Model file for the job. Use its own axes, mm. A direction names the side the tool comes from. Coordinates: 2 decimals unless noted, no trailing zeros. Order: outer loops, then holes, each group sorted by start corner. A loop starts at its lowest first (then second) coordinate and runs counter-clockwise, first axis right, second up.
from build123d import *

# Parameters (mm, degrees)
SKETCH_1_R      = 1.1
EXTRUDE_1_DEPTH = 3
EXTRUDE_2_DEPTH = 2


with BuildPart() as part:
    # 草图1 → 凸台-拉伸1 (new body)
    with BuildSketch(Plane.XY):
        with BuildLine():
            Line((-5, 5.5), (5, 5.5))
            ThreePointArc((5, 5.5), (10.5, 0), (5, -5.5))
            Line((5, -5.5), (-5, -5.5))
            ThreePointArc((-5, -5.5), (-10.5, 0), (-5, 5.5))
        make_face()
        Circle(SKETCH_1_R, mode=Mode.SUBTRACT)
    extrude(amount=EXTRUDE_1_DEPTH)

    # 草图3 → 凸台-拉伸2 (add)
    with BuildSketch(Plane(origin=(0, 0, 0), x_dir=(-1, 0, 0), z_dir=(0, 0, -1))):
        with BuildLine():
            Line((-1.802775638, 3), (-6.873863542, 3))
            ThreePointArc((-6.873863542, 3), (-7.154882442, 2.248923573), (-7.354101966, 1.472135955))
            Line((-7.354101966, 1.472135955), (-7.354101966, 1))
            Line((-7.354101966, 1), (-3.354101966, 1))
            ThreePointArc((-3.354101966, 1), (-2.765564437, 2.145146462), (-1.802775638, 3))
        make_face()
        with BuildLine():
            Line((-7.354101966, -1.472135955), (-7.354101966, -1))
            Line((-7.354101966, -1), (-3.354101966, -1))
            ThreePointArc((-3.354101966, -1), (-2.765564437, -2.145146462), (-1.802775638, -3))
            Line((-1.802775638, -3), (-6.873863542, -3))
            ThreePointArc((-6.873863542, -3), (-7.154882442, -2.248923573), (-7.354101966, -1.472135955))
        make_face()
        with BuildLine():
            Line((1.802775638, -3), (6.873863542, -3))
            ThreePointArc((6.873863542, -3), (7.154882442, -2.248923573), (7.354101966, -1.472135955))
            Line((7.354101966, -1.472135955), (7.354101966, -1))
            Line((7.354101966, -1), (3.354101966, -1))
            ThreePointArc((3.354101966, -1), (2.765564437, -2.145146462), (1.802775638, -3))
        make_face()
        with BuildLine():
            Line((7.354101966, 1.472135955), (7.354101966, 1))
            Line((7.354101966, 1), (3.354101966, 1))
            ThreePointArc((3.354101966, 1), (2.765564437, 2.145146462), (1.802775638, 3))
            Line((1.802775638, 3), (6.873863542, 3))
            ThreePointArc((6.873863542, 3), (7.154882442, 2.248923573), (7.354101966, 1.472135955))
        make_face()
    extrude(amount=EXTRUDE_2_DEPTH)


solid = part.part
Q1. Mould opens along X. For faces 1 (the face through (1.05, 0.33, 1.48)), 2 (the face through (2.8, 2.1, -1)), 3 (the face through (-10.5, -0.1, 1.5)), 4 (the face through (-5, -2, -2)) say: pulls with the +X half, pulls with the -X half, needs draft (parallel to the pull), parting line crosses it, or undercut.
Established:
face 1: undercut
face 2: undercut
face 3: pulls with the -X half
face 4: needs draft
Q2. Probe line 1 (Y direction, x = 4.75, z = -0.9); line 2 (Y direction, x = 0, z = 2.1); line 3 (Z direction, x = 1, y = 1.75). List the from-to ranges inside material, lowest first.
Established:
line 1: y = -3 to -1, 1 to 3
line 2: y = -5.5 to -1.1, 1.1 to 5.5
line 3: z = 0 to 3
Q3. Cut at D-D, the plane z = -0.55. List the corners of the cut face in (x, y).
Established:
outline: (-7.35, -1.47) arc R7.5 ccw to (-6.87, -3) - (-1.8, -3) arc R3.5 cw to (-3.35, -1) - (-7.35, -1) - close; (-7.35, 1) - (-3.35, 1) arc R3.5 cw to (-1.8, 3) - (-6.87, 3) arc R7.5 ccw to (-7.35, 1.47) - close; (1.8, -3) - (6.87, -3) arc R7.5 ccw to (7.35, -1.47) - (7.35, -1) - (3.35, -1) arc R3.5 cw to start; (1.8, 3) arc R3.5 cw to (3.35, 1) - (7.35, 1) - (7.35, 1.47) arc R7.5 ccw to (6.87, 3) - close
Q4. Cut at B-B, the plane x = 4.5. List the corners of the cut face in (y, z).
Established:
outline: (-5.5, 0) - (-3, 0) - (-3, -2) - (-1, -2) - (-1, 0) - (1, 0) - (1, -2) - (3, -2) - (3, 0) - (5.5, 0) - (5.5, 3) - (-5.5, 3) - close
Q5. Cut at C-C, the plane y = 0. List the corners of the cut face in (x, z), plus the area to 3 significant figures.
Established:
outline: (-10.5, 0) - (-1.1, 0) - (-1.1, 3) - (-10.5, 3) - close; (1.1, 0) - (10.5, 0) - (10.5, 3) - (1.1, 3) - close
area: 56.4 mm2
Q6. Which spindle directions (+Z, -Z, +X, -X, +Y, -Y) get a long thin tool onto all of the face, cutting with end or side? Do faces 5 (the face through (4, -3, -1)), 6 (the face through (-2.8, -2.1, -1)), 7 (the face through (7.15, -2.26, -0.99)), 8 (the face through (4, 3, -1)), 9 (the face through (-5, -1, -1)). Say none if no direction does.
Established:
face 5: -Z, +X, -X, -Y
face 6: -Z
face 7: -Z, +X, -Y
face 8: -Z, +X, -X, +Y
face 9: -Z, +X, -X
Q7. Drop flat-ended pins along their axis: P1, Ø1.6, axis at x = -5.5, z = -1, coming from the -Y side; P2, Ø0.6, axis at x = 5, z = -1.5, coming from the +Y side. Give the stop position or say it passes through.
Established:
P1: stops at y = -3
P2: stops at y = 3
Q8. Cut at A-A, the plane z = 1.45. List the corners of the cut face in (x, y), plus the area to 3 significant figures.
Established:
outline: (-5, -5.5) - (5, -5.5) arc R5.5 ccw to (5, 5.5) - (-5, 5.5) arc R5.5 ccw to start; hole circle Ø2.2 at (0, 0)
area: 201 mm2
